from build123d import *

# Parameters (mm, degrees)
SKETCH_1_W          = 100
SKETCH_1_H          = 80
EXTRUDE_1_DEPTH     = 2
SKETCH_3_R          = 1.35
CUT_EXTRUDE_1_DEPTH = 3
SKETCH_4_R          = 1.6
CUT_EXTRUDE_2_DEPTH = 3
SKETCH_5_R          = 1.6
CUT_EXTRUDE_3_DEPTH = 3
SKETCH_7_R          = 2.1
CUT_EXTRUDE_5_DEPTH = 10


with BuildPart() as part:
    # 草图1 → 凸台-拉伸1 (new body)
    with BuildSketch(Plane.XY):
        Rectangle(SKETCH_1_W, SKETCH_1_H)
    extrude(amount=EXTRUDE_1_DEPTH)

    # 草图3 → 切除-拉伸1 (cut, through all)
    with BuildSketch(Plane.XY.offset(2)):
        with Locations((-26.5, -24.5)):
            Circle(SKETCH_3_R)
        with Locations((-26.5, 24.5)):
            Circle(SKETCH_3_R)
        with Locations((31.5, 24.5)):
            Circle(SKETCH_3_R)
        with Locations((31.5, -24.5)):
            Circle(SKETCH_3_R)
    extrude(amount=-CUT_EXTRUDE_1_DEPTH, mode=Mode.SUBTRACT)

    # 草图4 → 切除-拉伸2 (cut, through all)
    with BuildSketch(Plane(origin=(0, 0, 0), x_dir=(-1, 0, 0), z_dir=(0, 0, -1))):
        with Locations((26.5, -36)):
            Circle(SKETCH_4_R)
    extrude(amount=-CUT_EXTRUDE_2_DEPTH, mode=Mode.SUBTRACT)

    # 草图5 → 切除-拉伸3 (cut, through all)
    with BuildSketch(Plane.XY.offset(2)):
        with Locations((-26.5, 36)):
            Circle(SKETCH_5_R)
    extrude(amount=-CUT_EXTRUDE_3_DEPTH, mode=Mode.SUBTRACT)

    # 草图7 → 切除-拉伸5 (cut)
    with BuildSketch(Plane.XY.offset(2)):
        with Locations((44, 17.5)):
            Circle(SKETCH_7_R)
        with Locations((44, -17.5)):
            Circle(SKETCH_7_R)
    extrude(amount=-CUT_EXTRUDE_5_DEPTH, mode=Mode.SUBTRACT)


solid = part.part
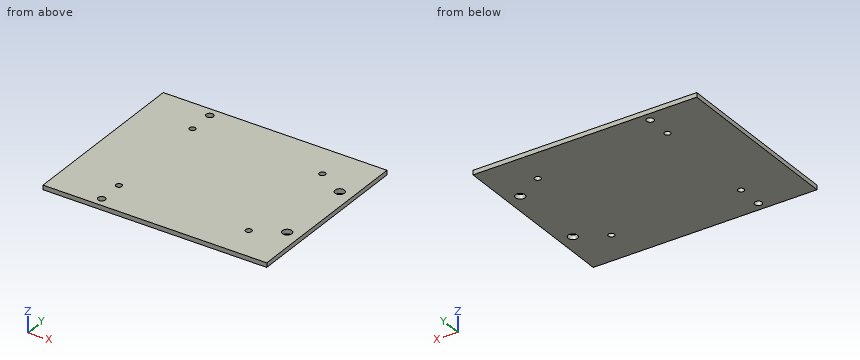
Could you check a few things on this model? Use its own coordinates, in mm. Give positions to 0.01 mm unless a question says otherwise; leave off trailing zeros. Order: outer loops, then holes, each group sorted by start corner. A loop starts at its lowest first (then second) coordinate and runs counter-clockwise, first axis right, second up. Notation, with made-up numbers: (-31.5, 74.25) - (-13.5, 74.25) arc R6 cw to (-13.5, 85.25) - close; hole circle Ø4 at (45.25, 29.5). An arc over 180 degrees is marked (long way). One line per item, written item: value. Start each with the question number.
1. Imagine slicing it at A-A on x = -26.5. List the corners of the cut face in (y, z) for me.
2. Imagine slicing it at B-B on y = 24.5. List the corners of the cut face in (x, z) for me, plus the area to 3 significant figures.
3. Imagine slicing it at D-D on y = 36. List the corners of the cut face in (x, z) for me, plus the area to 3 significant figures.
4. If I drill on probe 1 along Y at (x, z) = (-26.5, 0.55); probe 2 along Y at (x, z) = (44, 0.4); probe 3 along X at (y, z) = (16, 1.5), over which ranges is the centre line in solid material (lowest first)?
5. Imagine slicing it at C-C on x = 44. List the corners of the cut face in (y, z) for me.
Values:
1. outline: (-40, 0) - (-37.6, 0) - (-37.6, 2) - (-40, 2) - close; (-34.4, 0) - (-25.85, 0) - (-25.85, 2) - (-34.4, 2) - close; (-23.15, 0) - (23.15, 0) - (23.15, 2) - (-23.15, 2) - close; (25.85, 0) - (34.4, 0) - (34.4, 2) - (25.85, 2) - close; (37.6, 0) - (40, 0) - (40, 2) - (37.6, 2) - close
2. outline: (-50, 0) - (-27.85, 0) - (-27.85, 2) - (-50, 2) - close; (-25.15, 0) - (30.15, 0) - (30.15, 2) - (-25.15, 2) - close; (32.85, 0) - (50, 0) - (50, 2) - (32.85, 2) - close
2. area: 189 mm²
3. outline: (-50, 0) - (-28.1, 0) - (-28.1, 2) - (-50, 2) - close; (-24.9, 0) - (50, 0) - (50, 2) - (-24.9, 2) - close
3. area: 194 mm²
4. probe 1: -40 to -37.6, -34.4 to -25.85, -23.15 to 23.15, 25.85 to 34.4, 37.6 to 40
4. probe 2: -40 to -19.6, -15.4 to 15.4, 19.6 to 40
4. probe 3: -50 to 42.53, 45.47 to 50
5. outline: (-40, 0) - (-19.6, 0) - (-19.6, 2) - (-40, 2) - close; (-15.4, 0) - (15.4, 0) - (15.4, 2) - (-15.4, 2) - close; (19.6, 0) - (40, 0) - (40, 2) - (19.6, 2) - close
